Read the model definition and answer for the solid it produces. Units are mm, in the model's axes. A direction names the side the tool comes from. Coordinates: 2 decimals unless noted, no trailing zeros. Write each loop counter-clockwise with the first axis right and the second up, starting at its lowest first coordinate (ties: lowest second). Pieces come first, ordered by that corner, then holes.
(1) The mould has two halves that part along X. Classify faces 6 (the flat face through (-28, 3, -16.25)), 7 (the cylindrical face through (-21.086, 2.958, 16.515)), 8 (the cylindrical face through (-0.59, 7.1, -4.46)), 9 (the flat face through (-26, 3, 11.25)): +X half, -X half, draft (parallel to the pull), parting line (faces both ways), or undercut.
(2) Section C-C on y = -3.5 is taken. Write down the section's boundary in (x, z) (3 decimals), then the cut area to 3 significant figures.
(3) Find the intervals of material crossed by probe 1 along X at (y, z) = (4.5, 0); probe 2 along Y at (x, z) = (-10, -10); probe 3 along Y at (x, z) = (9, 23), in increasing order.
(4) Which of the six approach directions +Z, -Z, +X, -X, +Y, -Y give full straight-line access (tool end or side, diameter ignored) to faces 1 (the flat face through (-28, 3, 16.25)), 2 (the flat face through (-26, 3, -11.25)), 3 (the cylindrical face through (-7.493, 10.958, -0.33)), 4 (the flat face through (-6, -25, -21)), 5 (the cylindrical face through (-17.822, -24.65, -0.306))?
(5) Section A-A on y = -10 is taken. Write down the section's boundary in (x, z) (3 decimals), then the cut area to 3 significant figures.
(6) Section B-B on x = 0 is taken. Write down the section's boundary in (y, z), then the cut area to 3 significant figures.
(7) Section D-D on z = -2 is taken. State how many separate pieces and enclosed holes the cut face has, then the cut area to 3 significant figures.
(8) Given pin 1 (10 mm diameter, centred on x = -18, z = 19.5, fed in from -Y); pin 2 (12 mm diameter, centred on y = -34, z = -8.5, fed in from +X); pin 3 (6.5 mm diameter, centred on x = -23.5, y = 3.5, fed in from +Z); pin 4 (1 mm diameter, centred on x = -22, z = -8.5, fed in from +Y), each flat-ended and moving along its own axis, determine where each tip first touches the part or whether it passes through.
from build123d import *

# Parameters (mm, degrees)
BOSS_EXTRUDE4_DEPTH = 50
SKETCH7_R           = 1.75
CUT_EXTRUDE1_DEPTH  = 17.825
SKETCH8_R           = 0.75
SKETCH8_W           = 11.8
SKETCH8_H           = 22.5
BOSS_EXTRUDE5_DEPTH = 6
SKETCH9_R           = 7.5
BOSS_EXTRUDE6_DEPTH = 8
FILLET1_R           = 2
SKETCH10_R          = 4.5
CUT_EXTRUDE2_DEPTH  = 65


with BuildPart() as part:
    # Sketch6 → Boss-Extrude4 (new body)
    with BuildSketch(Plane.XZ):
        with BuildLine():
            Line((-1, 25.784833184), (-1, 12.785954208))
            ThreePointArc((-1, 12.785954208), (-12.825, 0), (-1, -12.785954208))
            Line((-1, -12.785954208), (-1, -25.784833184))
            Line((-1, -25.784833184), (-6, -25.784833184))
            Line((-6, -25.784833184), (-6, -16.784833184))
            ThreePointArc((-6, -16.784833184), (-17.825, 0), (-6, 16.784833184))
            Line((-6, 16.784833184), (-6, 25.784833184))
            Line((-6, 25.784833184), (-1, 25.784833184))
        make_face()
    extrude(amount=BOSS_EXTRUDE4_DEPTH)

    # Sketch7 → Cut-Extrude1 (cut, through all)
    with BuildSketch(Plane(origin=(-1, 0, 0), x_dir=(0, 0, -1), z_dir=(1, 0, 0))):
        with Locations((-19.285393696, -10)):
            Circle(SKETCH7_R)
        with Locations((-19.285393696, -40)):
            Circle(SKETCH7_R)
        with Locations((19.285393696, -40)):
            Circle(SKETCH7_R)
        with Locations((19.285393696, -10)):
            Circle(SKETCH7_R)
    extrude(amount=-CUT_EXTRUDE1_DEPTH, mode=Mode.SUBTRACT)

    # Sketch8 → Boss-Extrude5 (add)
    with BuildSketch(Plane(origin=(0, 0, 0), x_dir=(1, 0, 0), z_dir=(0, 1, 0))):
        with BuildLine():
            Line((-33.34361413, -16.25), (-22.318992281, -16.25))
            ThreePointArc((-22.318992281, -16.25), (-21.069616181, -16.522536094), (-20.047240136, -17.290627093))
            ThreePointArc((-20.047240136, -17.290627093), (26.473715688, 0), (-20.047240136, 17.290627093))
            ThreePointArc((-20.047240136, 17.290627093), (-21.069616181, 16.522536094), (-22.318992281, 16.25))
            Line((-22.318992281, 16.25), (-33.34361413, 16.25))
            ThreePointArc((-33.34361413, 16.25), (-35.464934474, 15.371320344), (-36.34361413, 13.25))
            Line((-36.34361413, 13.25), (-36.34361413, -13.25))
            ThreePointArc((-36.34361413, -13.25), (-35.464934474, -15.371320344), (-33.34361413, -16.25))
        make_face()
        with Locations((-25.44361413, 13.65)):
            Circle(SKETCH8_R, mode=Mode.SUBTRACT)
        with Locations((-25.44361413, -13.65)):
            Circle(SKETCH8_R, mode=Mode.SUBTRACT)
        with Locations((-25.44361413, 0)):
            Rectangle(SKETCH8_W, SKETCH8_H, mode=Mode.SUBTRACT)
    extrude(amount=BOSS_EXTRUDE5_DEPTH)

    # Sketch9 → Boss-Extrude6 (add)
    with BuildSketch(Plane(origin=(0, 6, 0), x_dir=(1, 0, 0), z_dir=(0, 1, 0))):
        Circle(SKETCH9_R)
    extrude(amount=BOSS_EXTRUDE6_DEPTH)

    # Fillet1
    fillet1_edges = [part.edges().sort_by_distance(p)[0] for p in [
        (-7.5, 6, 0),
    ]]
    fillet(fillet1_edges, radius=FILLET1_R)

    # Sketch10 → Cut-Extrude2 (cut, through all)
    with BuildSketch(Plane(origin=(0, 14, 0), x_dir=(1, 0, 0), z_dir=(0, 1, 0))):
        Circle(SKETCH10_R)
    extrude(amount=-CUT_EXTRUDE2_DEPTH, mode=Mode.SUBTRACT)


solid = part.part
Response:
1. face 6: draft
1. face 7: -X half
1. face 8: undercut
1. face 9: undercut
2. outline: (-6, -25.785) - (-1, -25.785) - (-1, -12.786) arc R12.825 cw to (-1, 12.786) - (-1, 25.785) - (-6, 25.785) - (-6, 16.785) arc R17.825 ccw to (-6, -16.785) - close
2. area: 314 mm2
3. probe 1: x = -36.34 to -31.34, -19.54 to -4.5, 4.5 to 26.47
3. probe 2: y = -50 to 6
3. probe 3: y = 0 to 6
4. face 1: +Z, -X, +Y, -Y
4. face 2: +Y, -Y
4. face 3: +Y
4. face 4: -Z, -X, -Y
4. face 5: -X, -Y
5. outline: (-6, -25.785) - (-1, -25.785) - (-1, -21.035) - (-6, -21.035) - close; (-6, -17.535) - (-1, -17.535) - (-1, -12.786) arc R12.825 cw to (-1, 12.786) - (-1, 17.535) - (-6, 17.535) - (-6, 16.785) arc R17.825 ccw to (-6, -16.785) - close; (-6, 21.035) - (-1, 21.035) - (-1, 25.785) - (-6, 25.785) - close
5. area: 279 mm2
6. outline: (0, -26.47) - (6, -26.47) - (6, -9.5) arc R2 cw to (8, -7.5) - (14, -7.5) - (14, -4.5) - (0, -4.5) - close; (0, 4.5) - (14, 4.5) - (14, 7.5) - (8, 7.5) arc R2 cw to (6, 9.5) - (6, 26.47) - (0, 26.47) - close
6. area: 313 mm2
7. separate pieces: 3
7. enclosed holes: 0
7. area: 562 mm2
8. pin 1: stops at y = 0
8. pin 2: stops at x = -1
8. pin 3: stops at z = 17.08
8. pin 4: passes through
